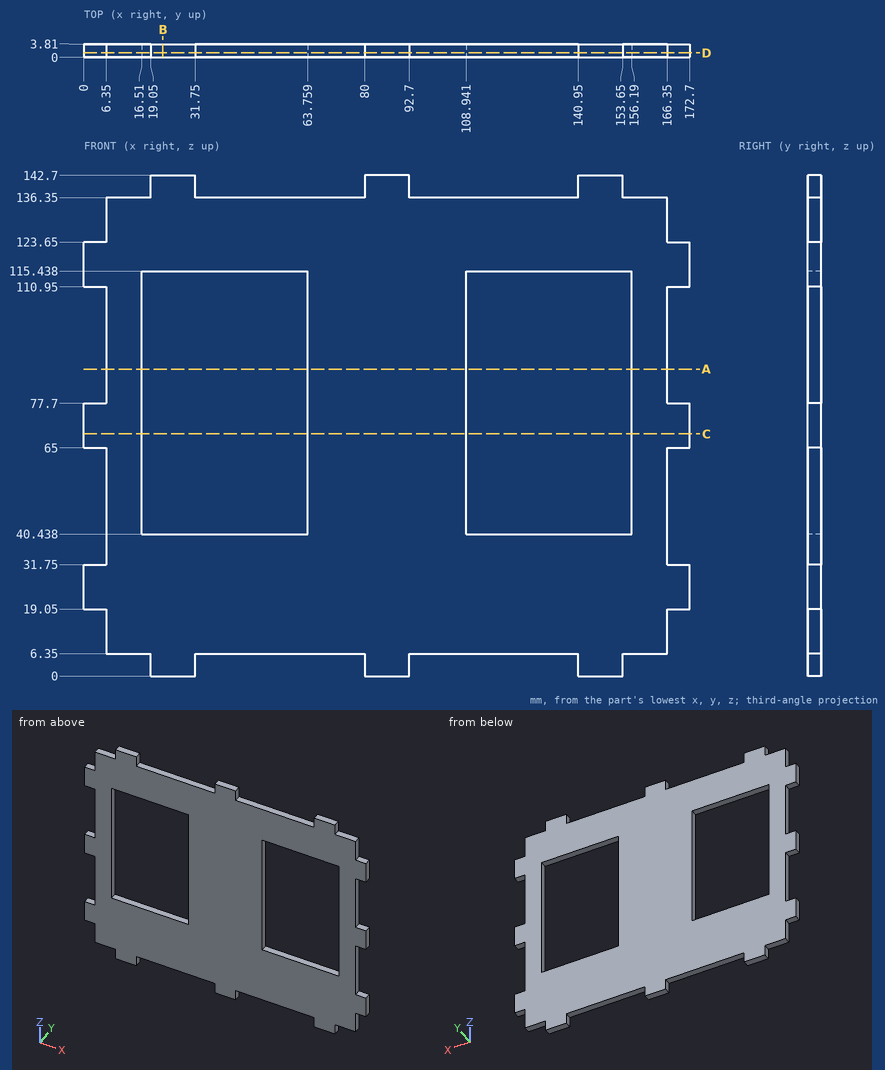
Verification items for this drawing (mm, ordinates from the low corner). Give positions to 0.01 mm unless a question says otherwise; leave off trailing zeros. Loops run counter-clockwise (first coordinate to the right, second up) from the corner with the lowest first, then second, coordinate; pieces in that order, holes last. Notation, with made-up numbers: M 4,12 L 31,12 A14 cw 31,37 Z; hole C -36.75,27 d4. An arc over 180 degrees is marked long. Answer as a JSON object with one key per item and string values. Group by question number.
Q1. Material ranges on line 1 along X through (y, z) = (2.6, 42.5); line 2 along Z through (x, y) = (116.5, 3.65), recorded low to high. Write a range as [from, to].
Q2. Cross-section at A-A on z = 87.5. Record the cut outline in (x, y).
Q3. Cross-section at D-D on y = 1.25. Give the number of separate pieces and of enclosed holes in the cut face, then the cut area to 3 significant figures.
Q4. Cross-section at B-B on x = 22.5. Record the cut outline in (y, z), then the cut area to 3 significant figures.
Q5. Cross-section at C-C on z = 69. Record the cut outline in (x, y).
Q6. Go/stop test with flat-tipped pins: P1, Ø1.9, axis at x = 123, y = 1, coming from the -Z side; P2, Ø2, axis at y = 1.5, z = 118, coming from the -X side; P3, Ø1.9, axis at y = 1, z = 139, coming from the -X side; P4, Ø1.5, axis at x = 120, y = 3, coming from the +Z side. Record where each tip stops, or that it passes through.
Evaluation:
{
 "1": {"line 1": "x = [6.35, 16.51], [63.76, 108.94], [156.19, 166.35]", "line 2": "z = [6.35, 40.44], [115.44, 136.35]"},
 "2": {"outline": "M 6.35,0 L 16.51,0 L 16.51,3.81 L 6.35,3.81 Z; M 63.76,0 L 108.94,0 L 108.94,3.81 L 63.76,3.81 Z; M 156.19,0 L 166.35,0 L 166.35,3.81 L 156.19,3.81 Z"},
 "3": {"separate pieces": "1", "enclosed holes": "2", "area": "14,700 mm2"},
 "4": {"outline": "M 0,0 L 3.81,0 L 3.81,40.44 L 0,40.44 Z; M 0,115.44 L 3.81,115.44 L 3.81,142.7 L 0,142.7 Z", "area": "258 mm2"},
 "5": {"outline": "M 0,0 L 16.51,0 L 16.51,3.81 L 0,3.81 Z; M 63.76,0 L 108.94,0 L 108.94,3.81 L 63.76,3.81 Z; M 156.19,0 L 172.7,0 L 172.7,3.81 L 156.19,3.81 Z"},
 "6": {"P1": "stops at z = 6.35", "P2": "stops at x = 0", "P3": "stops at x = 19.05", "P4": "stops at z = 136.35"}
}
